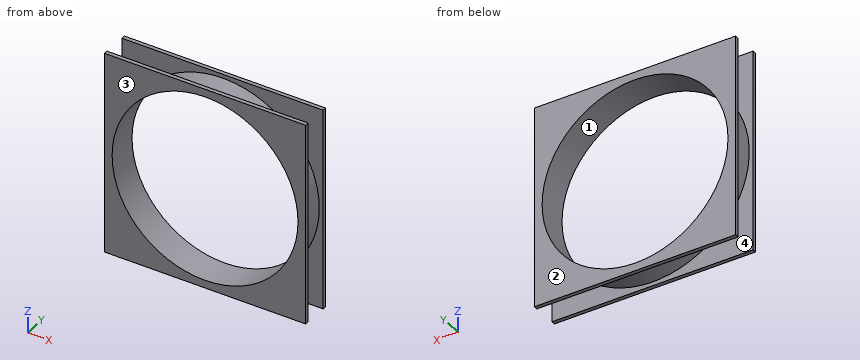
```python
from build123d import *

# Parameters (mm, degrees)
SKETCH1_R           = 62.5
SKETCH1_R_2         = 60
BOSS_EXTRUDE1_DEPTH = 7.5
SKETCH3_W           = 130
SKETCH3_H           = 130
SKETCH3_R           = 60
BOSS_EXTRUDE2_DEPTH = 2.5
SKETCH4_W           = 130
SKETCH4_H           = 130
SKETCH4_R           = 60
BOSS_EXTRUDE3_DEPTH = 2.5


with BuildPart() as part:
    # Sketch1 → Boss-Extrude1 (new body, symmetric)
    with BuildSketch(Plane(origin=(0, 0, 0), x_dir=(1, 0, 0), z_dir=(0, 1, 0))):
        Circle(SKETCH1_R)
        Circle(SKETCH1_R_2, mode=Mode.SUBTRACT)
    extrude(amount=BOSS_EXTRUDE1_DEPTH, both=True)

    # Sketch3 → Boss-Extrude2 (add)
    with BuildSketch(Plane(origin=(0, 7.5, 0), x_dir=(1, 0, 0), z_dir=(0, 1, 0))):
        Rectangle(SKETCH3_W, SKETCH3_H)
        Circle(SKETCH3_R, mode=Mode.SUBTRACT)
    extrude(amount=BOSS_EXTRUDE2_DEPTH)

    # Sketch4 → Boss-Extrude3 (add)
    with BuildSketch(Plane.XZ.offset(7.5)):
        Rectangle(SKETCH4_W, SKETCH4_H)
        Circle(SKETCH4_R, mode=Mode.SUBTRACT)
    extrude(amount=BOSS_EXTRUDE3_DEPTH)


solid = part.part
```
CAD build for the part. Positions are in the model's coordinates, mm. Face numbers are marked on the shaded views. A direction names the side the tool comes from. Give positions to 0.01 mm unless a question says otherwise; leave off trailing zeros. Order: outer loops, then holes, each group sorted by start corner. A loop starts at its lowest first (then second) coordinate and runs counter-clockwise, first axis right, second up. Notation, with made-up numbers: M 86.25,-6.75 L 98.25,-6.75 A36 ccw 98.25,28.25 Z; hole C -5,41.25 d3. An arc over 180 degrees is marked long. Put each result on its own line as item: value. Start each with the question number.
(1) Mould opens along Z. For the marked faces 1 and 2 say: +Z half, -Z half, draft (parallel to the pull), parting line (faces both ways), or undercut.
(2) Which spindle directions (+Z, -Z, +X, -X, +Y, -Y) get a long thin tool onto all of the face, cutting with end or side? Do the marked faces 3 and 4. Say none if no direction does.
(3) Saw through at C-C, the plane y = -1.75. Write the cut outline in (x, z).
(4) Saw through at A-A, the plane x = 0. Write the cut outline in (y, z), then the cut area to 3 significant figures.
(5) Drill centre lines: line 1 along Z through (x, y) = (0, -2.5); line 2 along Y through (x, z) = (-28.5, 57). Where is each one in solid material? Low to high.
(6) Saw through at B-B, the plane z = 0. Write the cut outline in (x, y).
(7) Flat gauge pins, fed straight in: pin 1 Ø2 at (y, z) = (-1, -13.5) entering from +X; pin 2 Ø12 at (x, y) = (9.5, -0.5) entering from +Z; pin 3 Ø5 at (x, y) = (16, 4) entering from -Z. Where does each tip first touch, or does it go through?
Check result:
1. face 1: undercut
1. face 2: draft
2. face 3: +Z, -Z, +X, -X, -Y
2. face 4: none
3. outline: C 0,0 d125; hole C 0,0 d120
4. outline: M -10,-65 L -7.5,-65 L -7.5,-62.5 L 7.5,-62.5 L 7.5,-65 L 10,-65 L 10,-60 L -10,-60 Z; M -10,60 L 10,60 L 10,65 L 7.5,65 L 7.5,62.5 L -7.5,62.5 L -7.5,65 L -10,65 Z
4. area: 125 mm2
5. line 1: z = -62.5 to -60, 60 to 62.5
5. line 2: y = -10 to -7.5, 7.5 to 10
6. outline: M -65,-10 L -60,-10 L -60,10 L -65,10 L -65,7.5 L -62.5,7.5 L -62.5,-7.5 L -65,-7.5 Z; M 60,-10 L 65,-10 L 65,-7.5 L 62.5,-7.5 L 62.5,7.5 L 65,7.5 L 65,10 L 60,10 Z
7. pin 1: stops at x = 61.24
7. pin 2: stops at z = 62.4
7. pin 3: stops at z = -61.02
